Model file for the job. Use its own axes, mm. Face numbers are marked on the shaded views. Round coordinates to 2 decimals unless told otherwise and drop trailing zeros. Loops run counter-clockwise (first coordinate to the right, second up) from the corner with the lowest first, then second, coordinate; pieces in that order, holes last. Notation, with made-up numbers: M -13.75,12.5 L 2.25,12.5 A29 ccw 2.25,38.5 Z; hole C 6.5,79 d4. An arc over 180 degrees is marked long. Use a Markdown table: item, result. Add a question column.
Item 1: Saw through at C-C on x = -3.25. Write the cut outline in (y, z), then the cut area to 3 significant figures.
Item 2: Two-plate mould, pull along Y, no slides. Class the marked faces 1 and 2: +Y half, -Y half, draft (parallel to the pull), parting line (faces both ways), or undercut.
Item 3: Pin check, flat tips, straight feed: P1, Ø3, axis at x = -3, y = 10, coming from the +Z side; P2, Ø1, axis at x = -0.5, y = 8.5, coming from the -Z side; P3, Ø8, axis at y = -9, z = 7.5, coming from the -X side; P4, Ø1.5, axis at x = -0.5, z = 0.5, coming from the +Y side. Stop position of each tip, or through.
Item 4: Wall check: L1, parallel to Y at x = -3.5, z = 0; L2, parallel to X at y = 10, z = 11.5; L3, parallel to Y at x = 2, z = -5. Give the ranges that are in metal, low to high. Write a range as from..to.
Item 5: Saw through at A-A on z = 0. Write the cut outline in (x, y).
Item 6: Saw through at D-D on x = 0. Write the cut outline in (y, z), then the cut area to 3 significant figures.
```python
from build123d import *

# Parameters (mm, degrees)
CUT_EXTRUDE1_START = -1
SKETCH3_R          = 15.5
SKETCH3_R_2        = 14.5
CUT_EXTRUDE1_DEPTH = 1


with BuildPart() as part:
    # Sketch2 → Revolve1 (revolve)
    with BuildSketch(Plane.XY, mode=Mode.PRIVATE) as revolve1_sk:
        with BuildLine():
            Line((-6, 14.5), (-2.449489743, 14.5))
            ThreePointArc((-2.449489743, 14.5), (0, 15.5), (2.449489743, 14.5))
            Line((2.449489743, 14.5), (6, 14.5))
            Line((6, 14.5), (6, 17))
            ThreePointArc((6, 17), (5.707106781, 17.707106781), (5, 18))
            Line((5, 18), (-5, 18))
            ThreePointArc((-5, 18), (-5.707106781, 17.707106781), (-6, 17))
            Line((-6, 17), (-6, 14.5))
        make_face()
    revolve(revolve1_sk.sketch.rotate(Axis((-6, 0, 0), (1, 0, 0)), 90), axis=Axis((-6, 0, 0), (1, 0, 0)))

    # Sketch3 → Cut-Extrude1 (cut)
    with BuildSketch(Plane.ZY.offset(6).offset(CUT_EXTRUDE1_START)):
        Circle(SKETCH3_R)
        Circle(SKETCH3_R_2, mode=Mode.SUBTRACT)
    cut_extrude1 = extrude(amount=CUT_EXTRUDE1_DEPTH, mode=Mode.SUBTRACT)

    # Mirror1: Cut-Extrude1 across plane
    add(cut_extrude1.mirror(Plane(origin=(0, 0, 0), x_dir=(0, 0, 1), z_dir=(1, 0, 0))), mode=Mode.SUBTRACT)


solid = part.part
```
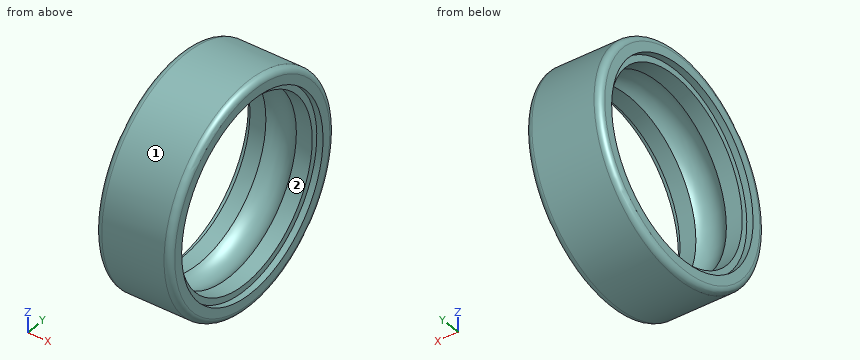
Entries:
| question | item | result |
|---|---|---|
| 1 | outline | C 0,0 d36; hole C 0,0 d29 |
| 1 | area | 357 mm2 |
| 2 | face 1 | parting line |
| 2 | face 2 | undercut |
| 3 | P1 | z = 15.87 |
| 3 | P2 | z = -16.12 |
| 3 | P3 | x = -6 |
| 3 | P4 | y = 18 |
| 4 | L1 | -18..-14.5, 14.5..18 |
| 4 | L2 | -5..-1.32, 1.32..5 |
| 4 | L3 | -17.29..-14.01, 14.01..17.29 |
| 5 | outline | M -6,-17 A1 ccw -5,-18 L 5,-18 A1 ccw 6,-17 L 6,-15.5 L 5,-15.5 L 5,-14.5 L 2.45,-14.5 A3.5 cw -2.45,-14.5 L -5,-14.5 L -5,-15.5 L -6,-15.5 Z; M -6,15.5 L -5,15.5 L -5,14.5 L -2.45,14.5 A3.5 cw 2.45,14.5 L 5,14.5 L 5,15.5 L 6,15.5 L 6,17 A1 ccw 5,18 L -5,18 A1 ccw -6,17 Z |
| 6 | outline | C 0,0 d36; hole C 0,0 d31 |
| 6 | area | 263 mm2 |
